from build123d import *

# Parameters (mm, degrees)
EXTRUDE_1_DEPTH           = 20
SKETCH_2_R                = 5.5
CUT_EXTRUDE_1_DEPTH       = 15
CUT_EXTRUDE_2_DEPTH       = 17
HOLE_WIZARD_M6_1_D        = 5
HOLE_WIZARD_1_D           = 5
HOLE_WIZARD_1_DEPTH       = 14
HOLE_WIZARD_1_CBORE_D     = 6
HOLE_WIZARD_1_CBORE_DEPTH = 1
HOLE_WIZARD_1_TIP         = 1.502151548


with BuildPart() as part:
    # 草图1 → 凸台-拉伸1 (new body)
    with BuildSketch(Plane.XY):
        Polygon((0, 0), (20, 0), (20, 1), (1, 20), (0, 20), align=None)
    extrude(amount=EXTRUDE_1_DEPTH)

    # 草图2 → 切除-拉伸1 (cut)
    with BuildSketch(Plane(origin=(0, 20, 0), x_dir=(1, 0, 0), z_dir=(0, 1, 0))):
        with Locations(Location((10, -10, 0), (0, 0, 270))):
            Circle(SKETCH_2_R)
    extrude(amount=-CUT_EXTRUDE_1_DEPTH, mode=Mode.SUBTRACT)

    # 草图3 → 切除-拉伸2 (cut)
    with BuildSketch(Plane(origin=(20, 0, 0), x_dir=(0, 0, -1), z_dir=(1, 0, 0))):
        with BuildLine():
            Line((-13.16227766, 5.5), (-6.83772234, 5.5))
            ThreePointArc((-6.83772234, 5.5), (-10, 15.5), (-13.16227766, 5.5))
        make_face()
    extrude(amount=-CUT_EXTRUDE_2_DEPTH, mode=Mode.SUBTRACT)

    # M6 螺纹孔1 (through all)
    with Locations(Plane(origin=(0, 5, 0), x_dir=(1, 0, 0), z_dir=(0, 1, 0))):
        with Locations((10, -10)):
            Hole(HOLE_WIZARD_M6_1_D / 2)

    # 打孔尺寸(%根据)内六角圆柱头螺钉的类型1
    with Locations(Plane(origin=(3, 0, 0), x_dir=(0, 0, -1), z_dir=(1, 0, 0))):
        with Locations((-10, 10)):
            CounterBoreHole(HOLE_WIZARD_1_D / 2, HOLE_WIZARD_1_CBORE_D / 2, HOLE_WIZARD_1_CBORE_DEPTH, depth=HOLE_WIZARD_1_DEPTH)
            with Locations((0, 0, -(HOLE_WIZARD_1_DEPTH + HOLE_WIZARD_1_TIP / 2))):  # 118° drill point
                Cone(0, HOLE_WIZARD_1_D / 2, HOLE_WIZARD_1_TIP, mode=Mode.SUBTRACT)


solid = part.part
Geometry: final body of the model. Coordinates: model frame, mm. A direction names the side the tool comes from. Give positions to 0.01 mm unless a question says otherwise; leave off trailing zeros. Write each loop counter-clockwise with the first axis right and the second up, starting at its lowest first coordinate (ties: lowest second). Pieces come first, ordered by that corner, then holes.
(1) Access query for faces 1 (the flat face through (8, 8, 20)), 2 (the flat face through (13, 5, 10)), 3 (the flat face through (4, 5.5, 10)), 4 (the flat face through (15.2, 5.5, 12.4)). Directions: +Z, -Z, +X, -X, +Y, -Y. A direction counts if a zero-diameter tool reaches every point of the face in a straight line with its end or side. Return the directions, or none.
(2) Cut plane C-C, the plane z = 17.25. Return loops of the section in (x, y).
(3) Cut plane D-D, the plane y = 13.75. Return loops of the section in (x, z).
(4) Mould query, pull axis Z, two halves, no side actions, for faces 5 (the flat face through (0, 12, 8)), 6 (the flat face through (15.3, 5.5, 7.6)), 7 (the flat face through (8, 8, 0)). Classes: released by +Z, released by -Z, zero draft, split by the parting line, or undercut.
(5) Cut plane A-A, the plane z = 11. Return loops of the section in (x, y), then the cut area to 3 significant figures.
(6) Cut plane B-B, the plane x = 16. Return loops of the section in (y, z), then the cut area to 3 significant figures.
(7) First-contact query: P1, Ø1, axis at y = 16, z = 16.5, coming from the +X side; P2, Ø4, axis at x = 8.5, z = 8.5, coming from the +Y side; P3, Ø4, axis at x = 6.5, z = 2, coming from the +Y side. Flat tips, straight axial feed; report the tip coordinate or a pass-through.
(8) Ray query, line 1 (Z direction, x = 4.75, y = 10); line 2 (Y direction, x = 14, z = 17); line 3 (X direction, y = 12.75, z = 10). Return the intervals inside material, ascending.
Values follow:
1. face 1: +Z, +X, -X, +Y, -Y
1. face 2: +Y
1. face 3: +X
1. face 4: +X, +Y
2. outline: (0, 0) - (20, 0) - (20, 1) - (1, 20) - (0, 20) - close
3. outline: (0, 0) - (7.25, 0) - (7.25, 5.24) arc R5.5 cw to (6.25, 5.98) - (3, 5.98) - (3, 14.02) - (6.25, 14.02) arc R5.5 cw to (7.25, 14.76) - (7.25, 20) - (0, 20) - close
4. face 5: zero draft
4. face 6: undercut
4. face 7: released by -Z
5. outline: (0, 0) - (7.71, 0) - (7.71, 5) - (4.59, 5) - (4.59, 5.5) - (3, 5.5) - (3, 7.17) - (2, 7.17) - (2, 7.71) - (0, 7.71) - close; (0, 12.29) - (2, 12.29) - (2, 12.83) - (3, 12.83) - (3, 15.41) - (4.59, 15.41) - (4.59, 16.41) - (1, 20) - (0, 20) - close; (12.29, 0) - (20, 0) - (20, 1) - (15.5, 5.5) - (15.41, 5.5) - (15.41, 5) - (12.29, 5) - close
5. area: 101 mm2
6. outline: (0, 0) - (5, 0) - (5, 20) - (0, 20) - close
6. area: 100 mm2
7. P1: stops at x = 5.5
7. P2: stops at y = 5
7. P3: stops at y = 16.5
8. line 1: z = 0 to 4.5, 15.5 to 20
8. line 2: y = 0 to 7
8. line 3: x = 0 to 2
